from build123d import *

# Parameters (mm, degrees)
F0_W     = 50.8
F0_H     = 50.8
F1_DEPTH = 50.8


with BuildPart() as f1:
    # F0 (on Top) → F1 (new body)
    with BuildSketch(Plane.XY):
        with BuildLine():
            ThreePointArc((609.6, 25.4), (579.842049, 97.242049), (508, 127))
            Line((508, 127), (-508, 127))
            ThreePointArc((-508, 127), (-579.842049, 97.242049), (-609.6, 25.4))
            Line((-609.6, 25.4), (-228.6, 25.4))
            Line((-228.6, 25.4), (-228.6, -25.4))
            Line((-228.6, -25.4), (-609.6, -25.4))
            ThreePointArc((-609.6, -25.4), (-579.842049, -97.242049), (-508, -127))
            Line((-508, -127), (508, -127))
            ThreePointArc((508, -127), (579.842049, -97.242049), (609.6, -25.4))
            Line((609.6, -25.4), (228.6, -25.4))
            Line((228.6, -25.4), (228.6, 25.4))
            Line((228.6, 25.4), (609.6, 25.4))
        make_face()
        Rectangle(F0_W, F0_H, mode=Mode.SUBTRACT)
    extrude(amount=F1_DEPTH)


solid = f1.part
Design review of the part built by this model. Coordinates are the model's own, in mm. A direction names the side the tool comes from. Give positions to 0.01 mm unless a question says otherwise; leave off trailing zeros. Loops run counter-clockwise (first coordinate to the right, second up) from the corner with the lowest first, then second, coordinate; pieces in that order, holes last. Notation, with made-up numbers: (54.25, -17) -> (90.25, -17) arc R11 cw to (90.25, -2) -> close; hole circle Ø2 at (5.25, 12.25). An arc over 180 degrees is marked (long way). One line per question, with ' | ' between items. Start each with the question number.
(1) We need section A-A (x = 409). State the section outline as (y, z) points, and give its area (3 significant figures).
(2) We need section C-C (y = 77). State the section outline as (x, z) points, and give its area (3 significant figures).
(3) For line 1 (Y direction, x = 491.5, z = 36); line 2 (X direction, y = 24, z = 36.5); line 3 (X direction, y = -25.5, z = 37), list the stretches that pass through material, from the lowest coordinate up.
(4) Insertion check: P1, Ø1.5, axis at y = 31.5, z = 16, coming from the +X side; P2, Ø10, axis at y = -13, z = 29.5, coming from the -X side. Each pin has a flat end and moves straight along its axis. Give the tip position at first contact, or say it passes through.
(5) Draft analysis for pull direction Y (two halves, no side actions). For faces 6 (the face through (580.628, 96.448, 25.044)), 7 (the face through (-422, 25.4, 25)), 8 (the face through (-9, 30, 50.8)), state which applies: +Y half, -Y half, draft (parallel to the pull), parting line (faces both ways), or undercut.
(6) We need section B-B (z = 36). State the section outline as (x, y) points.
(7) We need section D-D (y = -78). State the section outline as (x, z) points, and give its area (3 significant figures).
(8) For faces 1 (the face through (-579.048, 98.028, 25.044)), 2 (the face through (-580.628, -96.448, 25.044)), 3 (the face through (-416, -25.4, 25)), 4 (the face through (228.6, 0, 25)), 5 (the face through (0, 25.4, 25)), list the 3-axis set-ups (+Z, -Z, +X, -X, +Y, -Y) from which the entire face can be reached by the end or side of a thin tool; tool diameter is ignored.
The answers:
1) outline: (-127, 0) -> (-25.4, 0) -> (-25.4, 50.8) -> (-127, 50.8) -> close; (25.4, 0) -> (127, 0) -> (127, 50.8) -> (25.4, 50.8) -> close | area: 10,300 mm^2
2) outline: (-595.52, 0) -> (595.52, 0) -> (595.52, 50.8) -> (-595.52, 50.8) -> close | area: 60,500 mm^2
3) line 1: y = -127 to -25.4, 25.4 to 127 | line 2: x = -228.6 to -25.4, 25.4 to 228.6 | line 3: x = -609.6 to 609.6
4) P1: stops at x = 609.46 | P2: stops at x = -228.6
5) face 6: +Y half | face 7: undercut | face 8: draft
6) outline: (-609.6, -25.4) arc R101.6 ccw to (-508, -127) -> (508, -127) arc R101.6 ccw to (609.6, -25.4) -> (228.6, -25.4) -> (228.6, 25.4) -> (609.6, 25.4) arc R101.6 ccw to (508, 127) -> (-508, 127) arc R101.6 ccw to (-609.6, 25.4) -> (-228.6, 25.4) -> (-228.6, -25.4) -> close; hole (-25.4, -25.4) -> (25.4, -25.4) -> (25.4, 25.4) -> (-25.4, 25.4) -> close
7) outline: (-594.92, 0) -> (594.92, 0) -> (594.92, 50.8) -> (-594.92, 50.8) -> close | area: 60,400 mm^2
8) face 1: +Z, -Z, -X, +Y | face 2: +Z, -Z, -X, -Y | face 3: +Z, -Z, -X | face 4: +Z, -Z, +X | face 5: +Z, -Z
